```python
from build123d import *

# Parameters (mm, degrees)
SKETCH1_R               = 12.7
BOSS_EXTRUDE1_DEPTH     = 40
SKETCH2_R               = 37.5
BOSS_EXTRUDE2_DEPTH     = 2
SKETCH3_R               = 3.302
CUT_EXTRUDE1_DEPTH      = 43
SKETCH4_R               = 2.5
CUT_EXTRUDE2_DEPTH      = 38.5
CUT_EXTRUDE2_DEPTH_BACK = 38.5
SKETCH5_R               = 37.5
SKETCH5_R_2             = 12.7
BOSS_EXTRUDE3_DEPTH     = 1


with BuildPart() as part:
    # Sketch1 → Boss-Extrude1 (new body)
    with BuildSketch(Plane(origin=(0, 0, 0), x_dir=(1, 0, 0), z_dir=(0, 1, 0))):
        Circle(SKETCH1_R)
    extrude(amount=BOSS_EXTRUDE1_DEPTH)

    # Sketch2 → Boss-Extrude2 (add)
    with BuildSketch(Plane(origin=(0, 40, 0), x_dir=(1, 0, 0), z_dir=(0, 1, 0))):
        Circle(SKETCH2_R)
    extrude(amount=BOSS_EXTRUDE2_DEPTH)

    # Sketch3 → Cut-Extrude1 (cut, through all)
    with BuildSketch(Plane(origin=(0, 0, 0), x_dir=(-1, 0, 0), z_dir=(0, -1, 0))):
        Circle(SKETCH3_R)
    extrude(amount=-CUT_EXTRUDE1_DEPTH, mode=Mode.SUBTRACT)

    # Sketch4 → Cut-Extrude2 (cut, two sides)
    with BuildSketch(Plane.XY) as cut_extrude2_sk:
        with Locations((0, 20)):
            Circle(SKETCH4_R)
    extrude(amount=CUT_EXTRUDE2_DEPTH, mode=Mode.SUBTRACT)
    extrude(cut_extrude2_sk.sketch, amount=-CUT_EXTRUDE2_DEPTH_BACK, mode=Mode.SUBTRACT)

    # Sketch5 → Boss-Extrude3 (add)
    with BuildSketch(Plane.XZ.offset(-40)):
        Circle(SKETCH5_R)
        Circle(SKETCH5_R_2, mode=Mode.SUBTRACT)
    extrude(amount=BOSS_EXTRUDE3_DEPTH)


solid = part.part
```
Here's how the part is built. I have some questions about the finished solid (model axes, mm). A direction names the side the tool comes from. Give positions to 0.01 mm unless a question says otherwise; leave off trailing zeros. Write each loop counter-clockwise with the first axis right and the second up, starting at its lowest first coordinate (ties: lowest second). Pieces come first, ordered by that corner, then holes.
(1) If I drill on L1, parallel to X at y = 22.5, z = 0; L2, parallel to Y at x = 0, z = 6.75, over which ranges is the centre line in solid material (lowest first)?
Output values:
L1: x = -12.7 to -3.3, 3.3 to 12.7
L2: y = 0 to 17.5, 22.5 to 42
(2) Imagine slicing it at B-B, the plane z = 0. Write out the boundary of the cut face in (x, y), and give its area (3 significant figures).
Output values:
outline: (-37.5, 39) - (-12.7, 39) - (-12.7, 0) - (-3.3, 0) - (-3.3, 42) - (-37.5, 42) - close; (3.3, 0) - (12.7, 0) - (12.7, 39) - (37.5, 39) - (37.5, 42) - (3.3, 42) - close
area: 938 mm2
(3) Will these pins go through, and if not, where does the flat tip stop? pin 1 (1.5 mm diameter, centred on x = -4.5, y = 36, fed in from -Z); pin 2 (1 mm diameter, centred on x = 3, y = 12, fed in from +Z); pin 3 (4 mm diameter, centred on y = 16.5, z = -2, fed in from +X).
Output values:
pin 1: stops at z = -12.13
pin 2: stops at z = 12.45
pin 3: stops at x = 12.7
(4) Imagine slicing it at C-C, the plane y = 20. Write out the boundary of the cut face in (x, z).
Output values:
outline: (-2.5, -12.45) - (-2.5, -2.16) arc R3.3 cw to (-2.5, 2.16) - (-2.5, 12.45) arc R12.7 ccw to start; (2.5, -12.45) arc R12.7 ccw to (2.5, 12.45) - (2.5, 2.16) arc R3.3 cw to (2.5, -2.16) - close
(5) Imagine slicing it at A-A, the plane x = 0. Write out the boundary of the cut face in (y, z).
Output values:
outline: (0, -12.7) - (17.5, -12.7) - (17.5, -3.3) - (0, -3.3) - close; (0, 3.3) - (17.5, 3.3) - (17.5, 12.7) - (0, 12.7) - close; (22.5, -12.7) - (39, -12.7) - (39, -37.5) - (42, -37.5) - (42, -3.3) - (22.5, -3.3) - close; (22.5, 3.3) - (42, 3.3) - (42, 37.5) - (39, 37.5) - (39, 12.7) - (22.5, 12.7) - close
(6) On a 3-axis mill with a long thin cutter (end or side, diameter ignored), from which of +Z, -Z, +X, -X, +Y, -Y can I reach the whole of each face in a straight line? I mean faces 1 (the face through (-0.54, 17.56, -7.36)), 2 (the face through (16, 39, 1)). Say none if no direction works.
Output values:
face 1: +Z, -Z
face 2: -Y
(7) Thinking about a two-plate mould opening in Z: for faces 3 (the face through (3, 0, 3)), 4 (the face through (-2.75, 19.23, 12.4)), 5 (the face through (3.3, 20.7, -0.1)), which applies, pulls with the +Z half, pulls with the -Z half, needs draft (parallel to the pull), parting line crosses it, or undercut?
Output values:
face 3: needs draft
face 4: parting line crosses it
face 5: undercut
(8) Imagine slicing it at D-D, the plane y = 30.5. Write out the boundary of the cut face in (x, z).
Output values:
outline: circle Ø25.4 at (0, 0); hole circle Ø6.6 at (0, 0)
